CAD build for the part. Positions are in the model's coordinates, mm. A direction names the side the tool comes from. Round coordinates to 2 decimals unless told otherwise and drop trailing zeros. Order: outer loops, then holes, each group sorted by start corner. A loop starts at its lowest first (then second) coordinate and runs counter-clockwise, first axis right, second up. Notation, with made-up numbers: (-13.75, 14.25) - (7.25, 14.25) arc R15 ccw to (7.25, 30.25) - close; hole circle Ø9 at (12.5, 41.5). An arc over 180 degrees is marked (long way). Write item = value, one per line.
from build123d import *

# Parameters (mm, degrees)
SKETCH_W     = 6.3
SKETCH_H     = 6.3
PAD_DEPTH    = 10
SKETCH001_W  = 14
SKETCH001_H  = 14
PAD001_DEPTH = 2
SKETCH002_R  = 1.05
POCKET_DEPTH = 7.5
SKETCH003_W  = 6.3
SKETCH003_H  = 17.5
PAD002_DEPTH = 2
PAD003_DEPTH = 6.3
FILLET_R     = 0.4
FILLET001_R  = 0.4
CHAMFER_SIZE = 0.7


with BuildPart() as part:
    # Sketch → Pad (new body)
    with BuildSketch(Plane.XY):
        Rectangle(SKETCH_W, SKETCH_H)
    extrude(amount=PAD_DEPTH)

    # Sketch001 → Pad001 (join)
    with BuildSketch(Plane.XY):
        Rectangle(SKETCH001_W, SKETCH001_H)
    extrude(amount=-PAD001_DEPTH)

    # Sketch002 (on Face11 of Pad001) → Pocket (cut)
    with BuildSketch(Plane.XY.offset(10)):
        Circle(SKETCH002_R)
    extrude(amount=-POCKET_DEPTH, mode=Mode.SUBTRACT)

    # Sketch003 (on Face9 of Pocket) → Pad002 (join)
    with BuildSketch(Plane.YZ.offset(3.15)):
        with Locations((0, 8.75)):
            Rectangle(SKETCH003_W, SKETCH003_H)
    pad002 = extrude(amount=PAD002_DEPTH)

    # Sketch004 (on Face8 of Pad002) → Pad003 (join)
    with BuildSketch(Plane.XZ.offset(3.15)):
        Polygon((3.15, 17.5), (0.65, 16.5), (0.65, 15.5), (3.15, 12.5), align=None)
    pad003 = extrude(amount=-PAD003_DEPTH)

    # Mirrored: Pad003, Pad002 across Sketch004 V_Axis
    add(pad003.mirror(Plane(origin=(0, -3.15, 0), x_dir=(0, -1, 0), z_dir=(1, 0, 0))))
    add(pad002.mirror(Plane(origin=(0, -3.15, 0), x_dir=(0, -1, 0), z_dir=(1, 0, 0))))

    # Fillet
    fillet_edges = [part.edges().sort_by_distance(p)[0] for p in [
        (0.65, 0, 16.5),
    ]]
    fillet(fillet_edges, radius=FILLET_R)

    # Fillet001
    fillet001_edges = [part.edges().sort_by_distance(p)[0] for p in [
        (-0.65, 0, 16.5),
    ]]
    fillet(fillet001_edges, radius=FILLET001_R)

    # Chamfer
    chamfer_edges = [part.edges().sort_by_distance(p)[0] for p in [
        (-1.05, 0, 10),
    ]]
    chamfer(chamfer_edges, length=CHAMFER_SIZE)


solid = part.part
(1) Drop flat-ended pins along their axis: pin 1 (3 mm diameter, centred on y = -1.5, z = 6, fed in from -X); pin 2 (3 mm diameter, centred on x = 0, y = 0, fed in from +Z); pin 3 (8 mm diameter, centred on x = -3, z = 10, fed in from +Y). Give the stop position or say it passes through.
Solved:
pin_1 = -5.15
pin_2 = 16.84
pin_3 = 3.15
(2) Tool access for faces 4 (the flat face through (-1.9, 0, 14)), 5 (the flat face through (0, -3.15, 9)), 6 (the flat face through (2.041, -0.044, 17.057)): list every direction of +Z, -Z, +X, -X, +Y, -Y with a clear straight run to the whole face (end or side of a thin tool).
Solved:
face_4 = +Y, -Y
face_5 = +Z, +X, -X, -Y
face_6 = +Z, +Y, -Y
(3) Band-saw the part on C-C on y = 0. List the corners of the cut face in (x, z), plus the area to 3 significant figures.
Solved:
outline = (-7, -2) - (7, -2) - (7, 0) - (5.15, 0) - (5.15, 17.5) - (3.15, 17.5) - (0.9, 16.6) arc R0.4 ccw to (0.65, 16.23) - (0.65, 15.5) - (3.15, 12.5) - (3.15, 10) - (1.75, 10) - (1.05, 9.3) - (1.05, 2.5) - (-1.05, 2.5) - (-1.05, 9.3) - (-1.75, 10) - (-3.15, 10) - (-3.15, 12.5) - (-0.65, 15.5) - (-0.65, 16.23) arc R0.4 ccw to (-0.9, 16.6) - (-3.15, 17.5) - (-5.15, 17.5) - (-5.15, 0) - (-7, 0) - close
area = 160 mm²
(4) Band-saw the part on D-D on z = 6.25. List the corners of the cut face in (x, y).
Solved:
outline = (-5.15, -3.15) - (5.15, -3.15) - (5.15, 3.15) - (-5.15, 3.15) - close; hole circle Ø2.1 at (0, 0)
(5) Pull direction Y, two halves, no side cores. Call faces 1 (the flat face through (-3.15, 0, 11)), 2 (the cylindrical face through (1, 0.32, 5.95)), 3 (the flat face through (0, 3.15, 9)): released by +Y, released by -Y, zero draft, split by the parting line, or undercut.
Solved:
face_1 = zero draft
face_2 = undercut
face_3 = released by +Y
(6) Band-saw the part on B-B on x = 0. List the corners of the cut face in (y, z).
Solved:
outline = (-7, -2) - (7, -2) - (7, 0) - (3.15, 0) - (3.15, 10) - (1.75, 10) - (1.05, 9.3) - (1.05, 2.5) - (-1.05, 2.5) - (-1.05, 9.3) - (-1.75, 10) - (-3.15, 10) - (-3.15, 0) - (-7, 0) - close
(7) Probe line 1 along X through (y, z) = (-2.5, 11.75); line 2 along Y through (x, z) = (0, 5); line 3 along Z through (x, y) = (5.5, 5.25). List the from-to ranges inside material, lowest first.
Solved:
line_1 = -5.15 to -3.15, 3.15 to 5.15
line_2 = -3.15 to -1.05, 1.05 to 3.15
line_3 = -2 to 0
(8) Band-saw the part on A-A on z = 10.25. List the corners of the cut face in (x, y), plus the area to 3 significant figures.
Solved:
outline = (-5.15, -3.15) - (-3.15, -3.15) - (-3.15, 3.15) - (-5.15, 3.15) - close; (3.15, -3.15) - (5.15, -3.15) - (5.15, 3.15) - (3.15, 3.15) - close
area = 25.2 mm²
